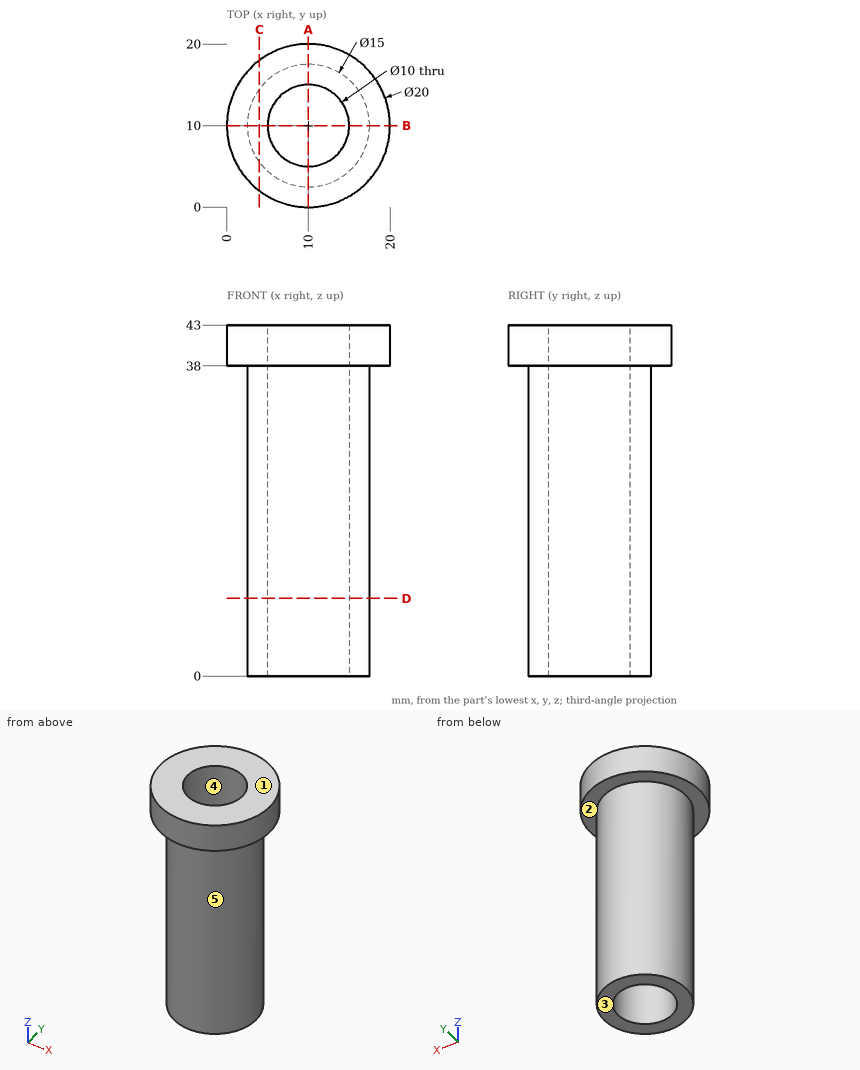
Input: dimensioned drawing with shaded views. Units: mm. Origin: part minimum x, y, z. A direction names the side the tool comes from. Coordinates: 2 decimals unless noted, no trailing zeros. Order: outer loops, then holes, each group sorted by start corner. A loop starts at its lowest first (then second) coordinate and runs counter-clockwise, first axis right, second up. Notation, with made-up numbers: M -8.5,-1.5 L 23.5,-1.5 A31 cw 23.5,37.5 Z; hole C 39.25,88 d1. An arc over 180 degrees is marked long. Answer as CSV lines item,"result".
Q1. Section C-C on x = 4. Return the cut outline in (y, z), and give its area (3 significant figures).
Answers:
outline,"M 2,38 L 5.5,38 L 5.5,0 L 14.5,0 L 14.5,38 L 18,38 L 18,43 L 2,43 Z"
area,"422 mm^2"
Q2. Line query: probe 1 along Y at (x, z) = (10, 30); probe 2 along Z at (x, y) = (1.25, 13); probe 3 along X at (y, z) = (13.25, 15). Output: solid intervals per line, ascending. Write a range as [from, to].
Answers:
probe 1,"y = [2.5, 5], [15, 17.5]"
probe 2,"z = [38, 43]"
probe 3,"x = [3.24, 6.2], [13.8, 16.76]"
Q3. Draft query along Y for the marked faces 3, 4 and 5. Return one class per face: pulls with the +Y half, pulls with the -Y half, needs draft (parallel to the pull), parting line crosses it, or undercut.
Answers:
face 3,"needs draft"
face 4,"undercut"
face 5,"parting line crosses it"
Q4. First-contact query: P1, Ø12, axis at y = 17, z = 38.5, coming from the -X side; P2, Ø6, axis at y = 12.5, z = 18.5, coming from the +X side; P3, Ø3, axis at x = 2.5, z = 38.5, coming from the +Y side. Flat tips, straight axial feed; report the tip coordinate or a pass-through.
Answers:
P1,"stops at x = 0.05"
P2,"stops at x = 17.5"
P3,"stops at y = 18"
Q5. Section D-D on z = 9.5. Return the cut outline in (x, y), and give its area (3 significant figures).
Answers:
outline,"C 10,10 d15; hole C 10,10 d10"
area,"98.2 mm^2"
Q6. Set-up query: the marked faces 1 and 2. Return all of +Z, -Z, +X, -X, +Y, -Y with unobstructed straight access to the full face (end or side cutting, diameter ignored); none if empty.
Answers:
face 1,"+Z, +X, -X, +Y, -Y"
face 2,"-Z"
Q7. Section A-A on x = 10. Return the cut outline in (y, z), and give its area (3 significant figures).
Answers:
outline,"M 0,38 L 2.5,38 L 2.5,0 L 5,0 L 5,43 L 0,43 Z; M 15,0 L 17.5,0 L 17.5,38 L 20,38 L 20,43 L 15,43 Z"
area,"240 mm^2"
